```python
from build123d import *

# Parameters (mm, degrees)
SKETCH1_R           = 22
BOSS_EXTRUDE1_DEPTH = 4
SKETCH2_R           = 31
BOSS_EXTRUDE2_DEPTH = 8
SKETCH3_R           = 1.5
CUT_EXTRUDE1_DEPTH  = 46.453272709
SKETCH4_R           = 18
BOSS_EXTRUDE3_DEPTH = 78
SKETCH5_R           = 17
CUT_EXTRUDE2_DEPTH  = 101.109939566
SKETCH6_R           = 20
SKETCH6_R_2         = 18
BOSS_EXTRUDE4_DEPTH = 4
LPATTERN1_COUNT     = 10
LPATTERN1_PITCH     = 8


with BuildPart() as part:
    # Sketch1 → Boss-Extrude1 (new body)
    with BuildSketch(Plane.XY):
        Circle(SKETCH1_R)
    extrude(amount=BOSS_EXTRUDE1_DEPTH)

    # Sketch2 → Boss-Extrude2 (add)
    with BuildSketch(Plane(origin=(0, 0, 0), x_dir=(-1, 0, 0), z_dir=(0, 0, -1))):
        Circle(SKETCH2_R)
    extrude(amount=BOSS_EXTRUDE2_DEPTH)

    # Sketch3 → Cut-Extrude1 (cut, through all)
    with BuildSketch(Plane(origin=(0, 0, -8), x_dir=(-1, 0, 0), z_dir=(0, 0, -1))):
        with Locations((-17.695427462, 16.213323131)):
            Circle(SKETCH3_R)
        with Locations((17.695427462, 16.213323131)):
            Circle(SKETCH3_R)
        with Locations((17.695427462, -16.213323131)):
            Circle(SKETCH3_R)
        with Locations((-17.695427462, -16.213323131)):
            Circle(SKETCH3_R)
    extrude(amount=-CUT_EXTRUDE1_DEPTH, mode=Mode.SUBTRACT)

    # Sketch4 → Boss-Extrude3 (add)
    with BuildSketch(Plane(origin=(0, 0, -8), x_dir=(-1, 0, 0), z_dir=(0, 0, -1))):
        Circle(SKETCH4_R)
    extrude(amount=BOSS_EXTRUDE3_DEPTH)

    # Sketch5 → Cut-Extrude2 (cut, through all)
    with BuildSketch(Plane(origin=(0, 0, -86), x_dir=(-1, 0, 0), z_dir=(0, 0, -1))):
        Circle(SKETCH5_R)
    extrude(amount=-CUT_EXTRUDE2_DEPTH, mode=Mode.SUBTRACT)

    # Sketch6 → Boss-Extrude4 (add)
    with BuildSketch(Plane(origin=(0, 0, -8), x_dir=(-1, 0, 0), z_dir=(0, 0, -1))):
        Circle(SKETCH6_R)
        Circle(SKETCH6_R_2, mode=Mode.SUBTRACT)
    boss_extrude4 = extrude(amount=BOSS_EXTRUDE4_DEPTH)

    # LPattern1: Boss-Extrude4 ×10
    with Locations(*[(0, 0, -i * LPATTERN1_PITCH) for i in range(1, LPATTERN1_COUNT)]):
        add(boss_extrude4)


solid = part.part
```
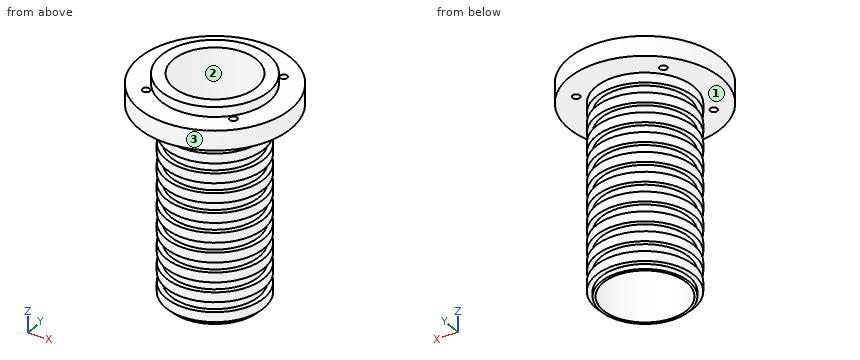
For this review, take the finished solid that the model builds, in its own axes (mm). Face numbers are marked on the shaded views. Coordinates: 2 decimals unless noted, no trailing zeros. Order: outer loops, then holes, each group sorted by start corner. A loop starts at its lowest first (then second) coordinate and runs counter-clockwise, first axis right, second up. Notation, with made-up numbers: (39, -1) - (71, -1) arc R30 cw to (71, 27) - close; hole circle Ø2 at (34.25, 58.25). An arc over 180 degrees is marked (long way). Answer as a JSON object with one key per item and string values. Group by question number.
1. We need section A-A on z = -38. State the section outline as (x, y) points, then the cut area to 3 significant figures.
2. For probe 1 along Y at (x, z) = (0, -38); probe 2 along X at (y, z) = (-15.5, -3); probe 3 along Y at (x, z) = (0, -50), list the stretches that pass through material, from the lowest coordinate up.
3. Clearance check with flat-ended pins moving along their axes: P1, Ø4, axis at x = 7, y = 23, coming from the +Z side; P2, Ø5, axis at x = 9, z = -56, coming from the -Y side; P3, Ø4, axis at x = -17.7, y = -16.21, coming from the -Z side. State where each tip first meets the part, or that it passes through.
4. The part is to be moulded in two halves that separate along X. For the marked faces 1, 2 and 3, say which applies: pulls with the +X half, pulls with the -X half, needs draft (parallel to the pull), parting line crosses it, or undercut.
5. We need section B-B on z = -2. State the section outline as (x, y) points.
Final values:
{
 "1": {"outline": "circle Ø36 at (0, 0); hole circle Ø34 at (0, 0)", "area": "110 mm²"},
 "2": {"probe 1": "-18 to -17, 17 to 18", "probe 2": "-26.85 to -19.01, -16.38 to -6.98, 6.98 to 16.38, 19.01 to 26.85", "probe 3": "-20 to -17, 17 to 20"},
 "3": {"P1": "z = 0", "P2": "y = -18.91", "P3": "z = -8"},
 "4": {"face 1": "needs draft", "face 2": "undercut", "face 3": "parting line crosses it"},
 "5": {"outline": "circle Ø62 at (0, 0); hole circle Ø3 at (-17.7, -16.21); hole circle Ø3 at (-17.7, 16.21); hole circle Ø34 at (0, 0); hole circle Ø3 at (17.7, -16.21); hole circle Ø3 at (17.7, 16.21)"}
}
